```python
from build123d import *

# Parameters (mm, degrees)
SKETCH2_W           = 30
SKETCH2_H           = 27
BOSS_EXTRUDE1_DEPTH = 20
SKETCH6_W           = 6.5
SKETCH6_H           = 26
CUT_EXTRUDE4_DEPTH  = 26
SKETCH9_W           = 5.5
SKETCH9_H           = 15
CUT_EXTRUDE5_DEPTH  = 21
SKETCH11_R          = 5
CUT_EXTRUDE8_DEPTH  = 0.5
SKETCH12_W          = 2.75
SKETCH12_H          = 11
CUT_EXTRUDE12_DEPTH = 17.5
SKETCH15_R          = 4.5
CUT_EXTRUDE13_DEPTH = 6


with BuildPart() as part:
    # Sketch2 → Boss-Extrude1 (new body)
    with BuildSketch(Plane(origin=(0, 0, 0), x_dir=(0, 0, -1), z_dir=(1, 0, 0))):
        with Locations((15, 13.5)):
            Rectangle(SKETCH2_W, SKETCH2_H)
    extrude(amount=BOSS_EXTRUDE1_DEPTH)

    # Sketch6 → Cut-Extrude4 (cut)
    with BuildSketch(Plane(origin=(2.296116437, 27, -0.293484995), x_dir=(1, 0, 0), z_dir=(0, 1, 0))):
        with Locations((12.115844825, 15.206515005)):
            Rectangle(SKETCH6_W, SKETCH6_H)
    extrude(amount=-CUT_EXTRUDE4_DEPTH, mode=Mode.SUBTRACT)

    # Sketch9 → Cut-Extrude5 (cut)
    with BuildSketch(Plane(origin=(0, 27, 0), x_dir=(1, 0, 0), z_dir=(0, 1, 0))):
        with Locations((8.411961261, 14)):
            Rectangle(SKETCH9_W, SKETCH9_H)
    extrude(amount=-CUT_EXTRUDE5_DEPTH, mode=Mode.SUBTRACT)

    # Sketch11 → Cut-Extrude8 (cut)
    with BuildSketch(Plane.ZY):
        with Locations((-15.1, 13.5)):
            Circle(SKETCH11_R)
    extrude(amount=-CUT_EXTRUDE8_DEPTH, mode=Mode.SUBTRACT)

    # Sketch12 → Cut-Extrude12 (cut)
    with BuildSketch(Plane(origin=(0, 27, 0), x_dir=(1, 0, 0), z_dir=(0, 1, 0))):
        with Locations((3.286961261, 15.5)):
            Rectangle(SKETCH12_W, SKETCH12_H)
    extrude(amount=-CUT_EXTRUDE12_DEPTH, mode=Mode.SUBTRACT)

    # Sketch15 → Cut-Extrude13 (cut)
    with BuildSketch(Plane.ZY.offset(-0.5)):
        with Locations((-15.04, 13.5)):
            Circle(SKETCH15_R)
    extrude(amount=-CUT_EXTRUDE13_DEPTH, mode=Mode.SUBTRACT)


solid = part.part
```
CAD build for the part. Positions are in the model's coordinates, mm. A direction names the side the tool comes from. Coordinates: 2 decimals unless noted, no trailing zeros. Write each loop counter-clockwise with the first axis right and the second up, starting at its lowest first coordinate (ties: lowest second). Pieces come first, ordered by that corner, then holes.
(1) Drill centre lines: probe 1 along Z at (x, y) = (4.25, 10); probe 2 along X at (y, z) = (3.5, -22.25); probe 3 along X at (y, z) = (23, -9.5). Where is each one in solid material? Low to high.
(2) Cut at B-B, the plane x = 13. List the corners of the cut face in (y, z).
(3) Cut at D-D, the plane z = -13.75. List the corners of the cut face in (x, y), and give its area (3 significant figures).
(4) Flat gauge pins, fed straight in: pin 1 (7 mm diameter, centred on x = 13.5, y = 8, fed in from +Z); pin 2 (5.5 mm diameter, centred on y = 13.5, z = -15.04, fed in from -X); pin 3 (3 mm diameter, centred on x = 14.5, z = -10.5, fed in from +Y). Where does each tip first touch, or does it go through?
(5) Two-plate mould, pull along Z, no slides. Class faces 4 (the face through (10, 0, -15)), 5 (the face through (8, 17, -21.5)), 6 (the face through (10, 13, 0)), 7 (the face through (17.662, 14, -15)): +Z half, -Z half, draft (parallel to the pull), parting line (faces both ways), or undercut.
(6) Cut at A-A, the plane y = 25.5. List the corners of the cut face in (x, z), and give its area (3 significant figures).
(7) Cut at C-C, the plane z = -25. List the corners of the cut face in (x, y).
(8) 3-axis set-ups, long thin cutter, end or side, ignore diameter. For faces 1 (the face through (20, 14, -15)), 2 (the face through (3, 18, -10)), 3 (the face through (3.04, 9.11, -16.02)): which of +Z, -Z, +X, -X, +Y, -Y reach the whole face in a straight line?
Geometry says:
1. probe 1: z = -30 to -21, -10 to 0
1. probe 2: x = 0 to 11.16, 17.66 to 20
1. probe 3: x = 0 to 5.66, 17.66 to 20
2. outline: (0, -30) - (27, -30) - (27, -28.5) - (1, -28.5) - (1, -2.5) - (27, -2.5) - (27, 0) - (0, 0) - close
3. outline: (0, 0) - (20, 0) - (20, 27) - (17.66, 27) - (17.66, 1) - (11.16, 1) - (11.16, 6) - (5.66, 6) - (5.66, 9.19) - (0.5, 9.19) - (0.5, 8.69) - (0, 8.69) - close; (0, 18.31) - (0.5, 18.31) - (0.5, 17.81) - (1.91, 17.81) - (1.91, 27) - (0, 27) - close; (4.66, 17.81) - (5.66, 17.81) - (5.66, 27) - (4.66, 27) - close
3. area: 181 mm2
4. pin 1: stops at z = 0
4. pin 2: stops at x = 17.66
4. pin 3: stops at y = 1
5. face 4: draft
5. face 5: undercut
5. face 6: +Z half
5. face 7: undercut
6. outline: (0, -30) - (20, -30) - (20, 0) - (0, 0) - close; hole (1.91, -21) - (4.66, -21) - (4.66, -10) - (1.91, -10) - close; hole (5.66, -21.5) - (11.16, -21.5) - (11.16, -28.5) - (17.66, -28.5) - (17.66, -2.5) - (11.16, -2.5) - (11.16, -6.5) - (5.66, -6.5) - close
6. area: 318 mm2
7. outline: (0, 0) - (20, 0) - (20, 27) - (17.66, 27) - (17.66, 1) - (11.16, 1) - (11.16, 27) - (0, 27) - close
8. face 1: +Z, -Z, +X, +Y, -Y
8. face 2: +Y
8. face 3: -X
